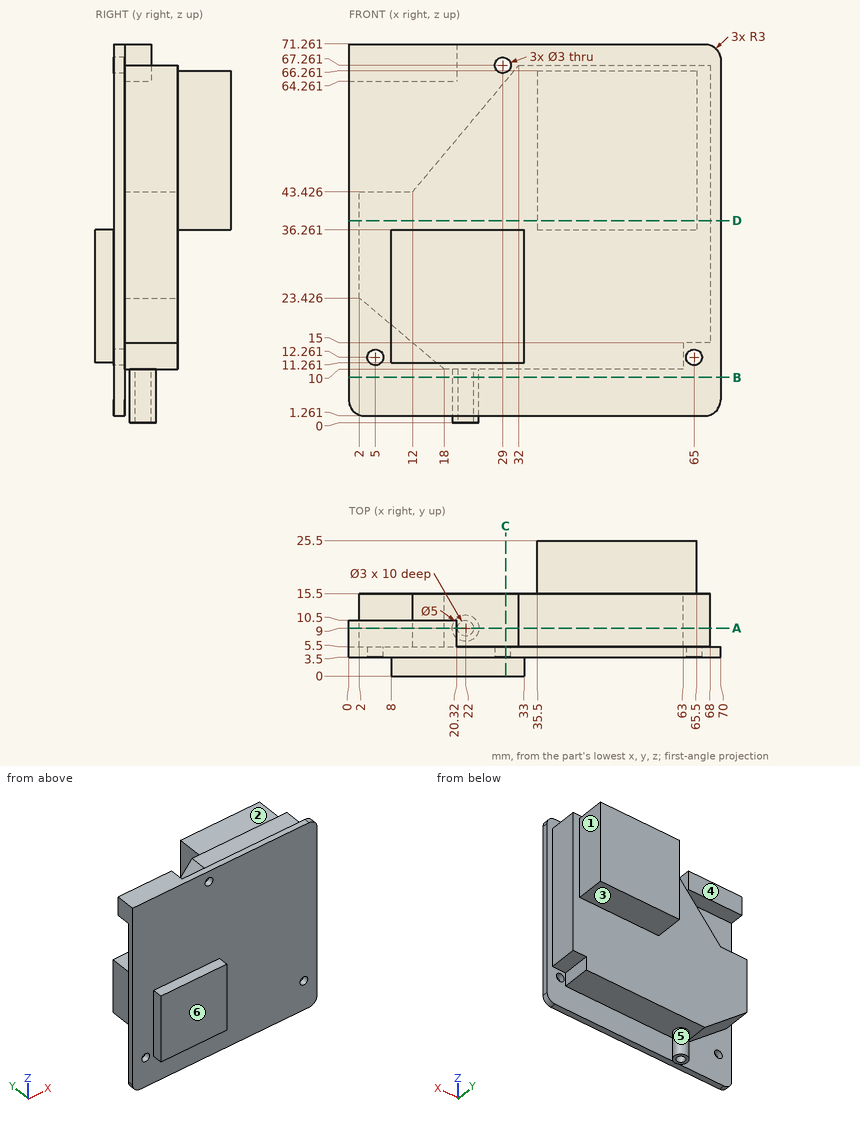
For this review, use the dimensioned drawing (mm, ordinates from the lowest corner) and the shaded views. A direction names the side the tool comes from. Round coordinates to 2 decimals unless told otherwise and drop trailing zeros. Order: outer loops, then holes, each group sorted by start corner. A loop starts at its lowest first (then second) coordinate and runs counter-clockwise, first axis right, second up.
1) Consider section C-C (x = 29.5). State the section outline as (y, z) points (1 decimal), plus the area to 3 significant figures.
The answers:
outline: (0, 11.3) - (3.5, 11.3) - (3.5, 1.3) - (5.5, 1.3) - (5.5, 10) - (15.5, 10) - (15.5, 64.3) - (5.5, 64.3) - (5.5, 65.8) - (3.5, 65.8) - (3.5, 36.3) - (0, 36.3) - close; (3.5, 68.7) - (5.5, 68.7) - (5.5, 71.3) - (3.5, 71.3) - close
area: 765 mm2
2) Consider section B-B (z = 8.5). State the section outline as (x, y) points.
The answers:
outline: (0, 3.5) - (70, 3.5) - (70, 5.5) - (0, 5.5) - close; circle Ø5 at (22, 9); hole circle Ø3 at (22, 9)
3) Clearance check with flat-ended pins moving along their axes: pin 1 Ø8 at (x, y) = (33, 8) entering from -Z; pin 2 Ø5 at (x, z) = (14.5, 47) entering from -Y; pin 3 Ø10 at (x, z) = (24, 32.5) entering from +Y. State where each tip first meets the part, or that it passes through.
The answers:
pin 1: stops at z = 1.26
pin 2: stops at y = 3.5
pin 3: stops at y = 15.5
4) Draft analysis for pull direction Y (two halves, no side actions). For the marked faces 4, 5 and 6, state which applies: released by +Y, released by -Y, zero draft, split by the parting line, or undercut.
The answers:
face 4: released by +Y
face 5: undercut
face 6: released by -Y
5) Machinability: for the marked faces 1, 2 and 3, which of the approach directions +Z, -Z, +X, -X, +Y, -Y give a long, thin tool a straight path to every point of the face, cutting with its end or side? Answer none if there is none.
The answers:
face 1: +Z, -Z, +X, +Y
face 2: +Z, +X, -X, +Y
face 3: -Z, +X, -X, +Y
6) Consider section A-A (y = 9). State the section outline as (x, z) points (1 decimal), plus the area to 3 significant figures.
The answers:
outline: (0, 64.3) - (20.3, 64.3) - (20.3, 71.3) - (0, 71.3) - close; (2, 23.4) - (18, 10) - (19.5, 10) - (19.5, 0) - (20.5, 0) - (20.5, 10) - (23.5, 10) - (23.5, 0) - (24.5, 0) - (24.5, 10) - (63, 10) - (63, 15) - (68, 15) - (68, 67.3) - (32, 67.3) - (12, 43.4) - (2, 43.4) - close
area: 3,330 mm2
7) For L1, parallel to Y at x = 22, z = 7; L2, parallel to Z at x = 5, y = 4.1; L3, parallel to X at y = 21.5, z = 44.5, list the stretches that pass through material, from the lowest coordinate up.
The answers:
L1: y = 3.5 to 5.5, 6.5 to 7.5, 10.5 to 11.5
L2: z = 1.26 to 10.76, 13.76 to 71.26
L3: x = 35.5 to 65.5
8) Consider section D-D (z = 38). State the section outline as (x, y) points.
The answers:
outline: (0, 3.5) - (70, 3.5) - (70, 5.5) - (68, 5.5) - (68, 15.5) - (65.5, 15.5) - (65.5, 25.5) - (35.5, 25.5) - (35.5, 15.5) - (2, 15.5) - (2, 5.5) - (0, 5.5) - close
